Check sheet for the modelled part. Datum: model origin and axes. Units: mm. Face numbers are marked on the shaded views. A direction names the side the tool comes from. Coordinates: 2 decimals unless noted, no trailing zeros. Loops run counter-clockwise (first coordinate to the right, second up) from the corner with the lowest first, then second, coordinate; pieces in that order, holes last. Notation, with made-up numbers: (-6, 14.25) - (22, 14.25) arc R37 ccw to (22, 53.25) - close; hole circle Ø7 at (77.5, 34.25). An arc over 180 degrees is marked (long way). Use a Markdown table: item, result. Add a question column.
1) Go/stop test with flat-tipped pins: P1, Ø1, axis at x = -3, y = 0.5, coming from the +Z side; P2, Ø1.5, axis at x = 7.5, y = 4, coming from the -Z side; P3, Ø1, axis at x = 5.5, y = 1, coming from the +Z side; P4, Ø3, axis at x = -0.5, y = -0.5, coming from the -Z side. Record where each tip stops, or that it passes through.
2) Thickness scan on line 1 (Y direction, x = 0, z = 3.65); line 2 (Y direction, x = 0, z = 19.5); line 3 (Z direction, x = -2, y = -7). Record the ranges inside material, lowest first.
3) Tool access check on the marked faces 4 and 5. Record the directions out of +Z, -Z, +X, -X, +Y, -Y that give a thin tool (end or side, any length) a straight path to the whole face; none if there is none.
4) Draft check along Y on the marked faces 1, 2 and 3. Enter one of: pulls with the +Y half, pulls with the -Y half, needs draft (parallel to the pull), parting line crosses it, or undercut.
5) Sectioned sample at A-A, the plane z = 28. Enter the section's corners in (x, y).
from build123d import *

# Parameters (mm, degrees)
F0_R     = 11
F1_DEPTH = 2
F2_R     = 5.5
F3_DEPTH = 4
F4_R     = 4
F5_DEPTH = 25
F6_R     = 2
F7_SIZE  = 1.99999
F8_T     = 2
F9_SIZE  = 3


# Not quite as in the source:
# - a fillet or chamfer is up to 0.001 mm smaller than in the source, because OpenCascade refuses the exact size
# - a shell that OpenCascade refuses in one call is made with other operations: the cavity is built on its own and cut out


with BuildPart() as f1:
    # F0 (on Top) → F1 (new body)
    with BuildSketch(Plane.XY):
        Circle(F0_R)
    extrude(amount=F1_DEPTH)

    # F2 (on face) → F3 (join)
    with BuildSketch(Plane.XY.offset(2)):
        Circle(F2_R)
    extrude(amount=F3_DEPTH)

    # F4 (on face) → F5 (join)
    with BuildSketch(Plane.XY.offset(6)):
        Circle(F4_R)
    extrude(amount=F5_DEPTH)

    # F6
    f6_edges = [f1.edges().sort_by_distance(p)[0] for p in [
        (-4, 0, 31),
    ]]
    fillet(f6_edges, radius=F6_R)

    # F7 (size 2 in the source; OpenCascade refuses exactly that, so slightly less here)
    f7_edges = [f1.edges().sort_by_distance(p)[0] for p in [
        (-11, 0, 2),
    ]]
    chamfer(f7_edges, length=F7_SIZE)

    # F8: shell of thickness 2, made by hand


with BuildPart() as f8_core1:
    # F8_t2: copy of F1
    add(f1.part)

    # the walls: a layer under each face that stays
    f8_faces = [f8_core1.faces().sort_by_distance(p)[0] for p in [
        (-6.0000066667, -6.0000066667, 2),
        (-10.000005, 0, 1.000005),
        (-5.5, 0, 4),
        (-11, 0, 5e-06),
        (-3.6666666667, -3.6666666667, 6),
        (-4, 0, 17.5),
        (0, 0, 31),
    ]]
    thicken(f8_faces, amount=-F8_T, mode=Mode.SUBTRACT)

    # F8_s3 → F8_t4 (revolve, cut)
    with BuildSketch(Plane.XZ):
        Polygon((5.52, 2.02), (5.5, 0), (3.5, 0), (3.5, 2), align=None)
    revolve(axis=Axis((0, 0, 2), (0, 0, 1)), mode=Mode.SUBTRACT)

    # F8_s5 → F8_t6 (revolve, cut)
    with BuildSketch(Plane.XZ):
        Polygon((4.02, 6.02), (4, 4), (2, 4), (2, 6), align=None)
    revolve(axis=Axis((0, 0, 6), (0, 0, 1)), mode=Mode.SUBTRACT)


with BuildPart() as f1_1:
    add(f1.part)

    # what is left inside the walls is the cavity
    f8_cavity = [f8_core1.part.solids().sort_by_distance(p)[0] for p in [
        (-1.98, 0, 12.333333),
    ]]
    add(f8_cavity, mode=Mode.SUBTRACT)

    # F9
    f9_edges = [f1_1.edges().sort_by_distance(p)[0] for p in [
        (-3.5, 0, 0),
    ]]
    chamfer(f9_edges, length=F9_SIZE)


solid = f1_1.part
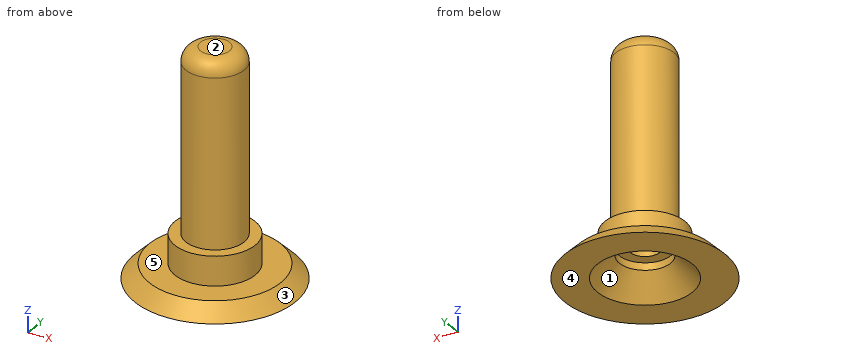
Solved:
| question | item | result |
|---|---|---|
| 1 | P1 | stops at z = 30.93 |
| 1 | P2 | stops at z = 0 |
| 1 | P3 | stops at z = 6 |
| 1 | P4 | stops at z = 4 |
| 2 | line 1 | y = -5.5 to -3.5, 3.5 to 5.5 |
| 2 | line 2 | y = -4 to -2, 2 to 4 |
| 2 | line 3 | z = 0 to 2 |
| 3 | face 4 | -Z, +X, -X, +Y, -Y |
| 3 | face 5 | +Z |
| 4 | face 1 | undercut |
| 4 | face 2 | needs draft |
| 4 | face 3 | parting line crosses it |
| 5 | outline | circle Ø8 at (0, 0); hole circle Ø4 at (0, 0) |
